Work out the finished part from the listing and answer in its coordinate system (mm). Round coordinates to 2 decimals unless told otherwise and drop trailing zeros. Loops run counter-clockwise (first coordinate to the right, second up) from the corner with the lowest first, then second, coordinate; pieces in that order, holes last.
```python
from build123d import *

# Parameters (mm, degrees)
F0_R     = 4.58
F0_R_2   = 11
F1_DEPTH = 3


with BuildPart() as f1:
    # F0 (on Top) → F1 (new body)
    with BuildSketch(Plane.XY):
        Polygon((-10.3433931154, -17.9152823985), (10.3433931154, -17.9152823985), (32.1102169209, -0.2177119583), (23.3435776075, -41.0728769962), (47.241943689, -0.3203072748), (16.2436525471, 27.6994075954), (20.6867862307, 0), (10.3433931154, 17.9152823985), (-15.8665643739, 27.9171195537), (23.8983660815, 40.7525697215), (-23.3435776075, 41.0728769962), (-32.1102169209, 0.2177119583), (-10.3433931154, 17.9152823985), (-20.6867862307, 0), (-16.2436525471, -27.6994075954), (-47.241943689, 0.3203072748), (-23.8983660815, -40.7525697215), (15.8665643739, -27.9171195537), align=None)
        with Locations((-21.741848439, -31.328804791)):
            Circle(F0_R, mode=Mode.SUBTRACT)
        with Locations((-8.1714619327, -27.0660405942)):
            Circle(F0_R, mode=Mode.SUBTRACT)
        Circle(F0_R_2, mode=Mode.SUBTRACT)
        with Locations((38.0024650387, -3.1645906779)):
            Circle(F0_R, mode=Mode.SUBTRACT)
        with Locations((-19.3541477681, 20.6097139168)):
            Circle(F0_R, mode=Mode.SUBTRACT)
        with Locations((-16.2606165997, 34.4933954689)):
            Circle(F0_R, mode=Mode.SUBTRACT)
        with Locations((27.5256097008, 6.4563266774)):
            Circle(F0_R, mode=Mode.SUBTRACT)
    extrude(amount=F1_DEPTH)


solid = f1.part
```
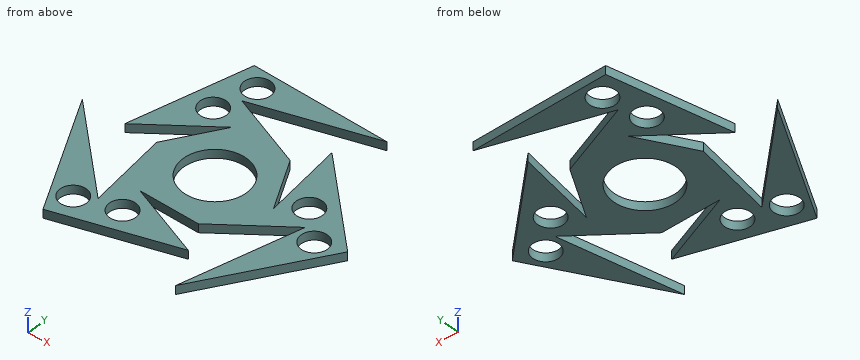
1. Find section A-A (y = -25.5). Write down the section's boundary in (x, z).
Answer key:
outline: (-32.57, 0) - (-18.68, 0) - (-18.68, 3) - (-32.57, 3) - close; (-16.6, 0) - (-12.48, 0) - (-12.48, 3) - (-16.6, 3) - close; (-3.87, 0) - (9.53, 0) - (9.53, 3) - (-3.87, 3) - close; (26.69, 0) - (32.48, 0) - (32.48, 3) - (26.69, 3) - close
2. Consider probe 1 along Y at (x, z) = (-6, 1.6); probe 2 along X at (y, z) = (-2.5, 1.9); probe 3 along Y at (x, z) = (12, 0.7). Determine where each line is inside the solid, lowest interval first.
Answer key:
probe 1: y = -34.98 to -31.1, -23.03 to -19.57, -17.92 to -9.22, 9.22 to 24.15, 31.1 to 40.96
probe 2: x = -45.64 to -44.12, -20.29 to -10.71, 10.71 to 29.3, 31.62 to 33.47, 42.53 to 45.96
probe 3: y = -29.17 to -26.44, -16.57 to 15.05, 36.91 to 40.83
3. Given pin 1 (1.5 mm diameter, centred on x = -1.5, z = 2.5, fed in from -Y); pin 2 (1.5 mm diameter, centred on x = -3.5, z = 1.5, fed in from -Y); pin 3 (1 mm diameter, centred on y = -20.5, z = 1.5, fed in from +X), each flat-ended and moving along its own axis, determine where each tip first touches the part or whether it passes through.
Answer key:
pin 1: stops at y = -33.76
pin 2: stops at y = -34.41
pin 3: stops at x = 35.7
4. Find section D-D (x = 30). Write down the section's boundary in (y, z), then the cut area to 3 significant figures.
Answer key:
outline: (-29.72, 0) - (-10.05, 0) - (-10.05, 3) - (-29.72, 3) - close; (-1.93, 0) - (2.6, 0) - (2.6, 3) - (-1.93, 3) - close; (10.31, 0) - (15.26, 0) - (15.26, 3) - (10.31, 3) - close
area: 87.5 mm2
5. Find section C-C (x = -19). Write down the section's boundary in (y, z).
Answer key:
outline: (-39.17, 0) - (-35, 0) - (-35, 3) - (-39.17, 3) - close; (-27.66, 0) - (-25.21, 0) - (-25.21, 3) - (-27.66, 3) - close; (-10.52, 0) - (2.92, 0) - (2.92, 3) - (-10.52, 3) - close; (10.88, 0) - (16.04, 0) - (16.04, 3) - (10.88, 3) - close; (25.18, 0) - (30.82, 0) - (30.82, 3) - (25.18, 3) - close; (38.16, 0) - (41.04, 0) - (41.04, 3) - (38.16, 3) - close
6. Find section B-B (z = 1.85). Write down the section's boundary in (x, y), then the cut area to 3 significant figures.
Answer key:
outline: (-47.24, 0.32) - (-23.9, -40.75) - (15.87, -27.92) - (-10.34, -17.92) - (10.34, -17.92) - (32.11, -0.22) - (23.34, -41.07) - (47.24, -0.32) - (16.24, 27.7) - (20.69, 0) - (10.34, 17.92) - (-15.87, 27.92) - (23.9, 40.75) - (-23.34, 41.07) - (-32.11, 0.22) - (-10.34, 17.92) - (-20.69, 0) - (-16.24, -27.7) - close; hole circle Ø9.16 at (-21.74, -31.33); hole circle Ø9.16 at (-19.35, 20.61); hole circle Ø9.16 at (-16.26, 34.49); hole circle Ø9.16 at (-8.17, -27.07); hole circle Ø22 at (0, 0); hole circle Ø9.16 at (27.53, 6.46); hole circle Ø9.16 at (38, -3.16)
area: 2,680 mm2
